```python
from build123d import *

# Parameters (mm, degrees)
BOSS_EXTRUDE1_DEPTH = 12.7
SKETCH3_W           = 25.4
SKETCH3_H           = 2.794
CUT_EXTRUDE1_DEPTH  = 9.525


with BuildPart() as part:
    # Sketch2 → Boss-Extrude1 (new body)
    with BuildSketch(Plane(origin=(0, 0, 0), x_dir=(1, 0, 0), z_dir=(0, 1, 0))):
        Polygon((-4.572, 0), (-12.7, 0), (-12.7, -9.525), (12.7, -9.525), (12.7, 0), (4.572, 0), (4.572, 12.7), (1.397, 12.7), (1.397, -3.3655), (-1.397, -3.3655), (-1.397, 12.7), (-4.572, 12.7), align=None)
    extrude(amount=BOSS_EXTRUDE1_DEPTH)

    # Sketch3 → Cut-Extrude1 (cut)
    with BuildSketch(Plane.XZ):
        with Locations((0, 4.7625)):
            Rectangle(SKETCH3_W, SKETCH3_H)
    extrude(amount=-CUT_EXTRUDE1_DEPTH, mode=Mode.SUBTRACT)


solid = part.part
```
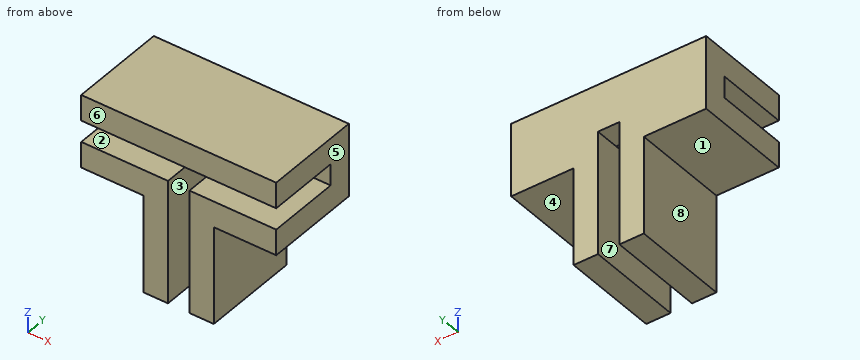
Geometry check sheet. Reference: the model listing, model coordinates, mm. Face numbers are marked on the shaded views. A direction names the side the tool comes from. Coordinates: 2 decimals unless noted, no trailing zeros. Write each loop counter-clockwise with the first axis right and the second up, starting at its lowest first coordinate (ties: lowest second). Pieces come first, ordered by that corner, then holes. Notation, with made-up numbers: M 44,35 L 64,35 A9 cw 64,52 Z; hole C -25.5,21 d8. An arc over 180 degrees is marked long. Use one line per item in the form item = value. Start each with the question number.
1) Section check C-C on x = -3. Enter the section's corners in (y, z) (1 decimal), and give its area (3 significant figures).
2) Thickness scan on probe 1 along X at (y, z) = (5.25, -8.25); probe 2 along X at (y, z) = (7.75, 0.25); probe 3 along Z at (x, y) = (8.5, 5) (1 decimal). Record the ranges inside material, lowest first. Write a range as from..to.
3) Go/stop test with flat-tipped pins: pin 1 Ø1.5 at (y, z) = (3.5, -4.5) entering from -X; pin 2 Ø3 at (x, z) = (-9.5, -1) entering from +Y; pin 3 Ø0.8 at (x, y) = (0.5, 10.5) entering from -Z; pin 4 Ø4 at (x, y) = (7, 7) entering from -Z. Record where each tip stops, or that it passes through.
4) Section check A-A on y = 4. Enter the section's corners in (x, z) (1 decimal), and give its area (3 significant figures).
5) Set-up check for the marked faces 1, 2, 3, 4 and 5: record each of +Z, -Z, +X, -X, +Y, -Y from which the full face is reachable in a straight line by a thin tool's end or side.
6) Section check B-B on z = -6.25. Enter the section's corners in (x, y).
7) Section check D-D on x = -10.5. Enter the section's corners in (y, z) (1 decimal), and give its area (3 significant figures).
8) Release check for a two-part mould opening along X. For the marked faces 6, 7 and 8 record: pulls with the +X half, pulls with the -X half, needs draft (parallel to the pull), parting line crosses it, or undercut.
Responses:
q1.outline = M 0,-12.7 L 12.7,-12.7 L 12.7,9.5 L 0,9.5 L 0,6.2 L 9.5,6.2 L 9.5,3.4 L 0,3.4 Z
q1.area = 256 mm2
q2.probe_1 = -4.57..-1.4, 1.4..4.57
q2.probe_2 = -12.7..-1.4, 1.4..12.7
q2.probe_3 = 0..3.4, 6.2..9.5
q3.pin_1 = -4.57
q3.pin_2 = 12.7
q3.pin_3 = 3.37
q3.pin_4 = 0
q4.outline = M -12.7,0 L -4.6,0 L -4.6,-12.7 L -1.4,-12.7 L -1.4,3.4 L -12.7,3.4 Z; M -12.7,6.2 L 12.7,6.2 L 12.7,9.5 L -12.7,9.5 Z; M 1.4,-12.7 L 4.6,-12.7 L 4.6,0 L 12.7,0 L 12.7,3.4 L 1.4,3.4 Z
q4.area = 242 mm2
q5.face_1 = -Z, -X, +Y, -Y
q5.face_2 = +X, -X, -Y
q5.face_3 = -Z, +Y, -Y
q5.face_4 = -Z, +X, +Y, -Y
q5.face_5 = +Z, -Z, +X, +Y, -Y
q6.outline = M -4.57,0 L -1.4,0 L -1.4,12.7 L -4.57,12.7 Z; M 1.4,0 L 4.57,0 L 4.57,12.7 L 1.4,12.7 Z
q7.outline = M 0,0 L 12.7,0 L 12.7,9.5 L 0,9.5 L 0,6.2 L 9.5,6.2 L 9.5,3.4 L 0,3.4 Z
q7.area = 94.4 mm2
q8.face_6 = needs draft
q8.face_7 = undercut
q8.face_8 = pulls with the -X half
